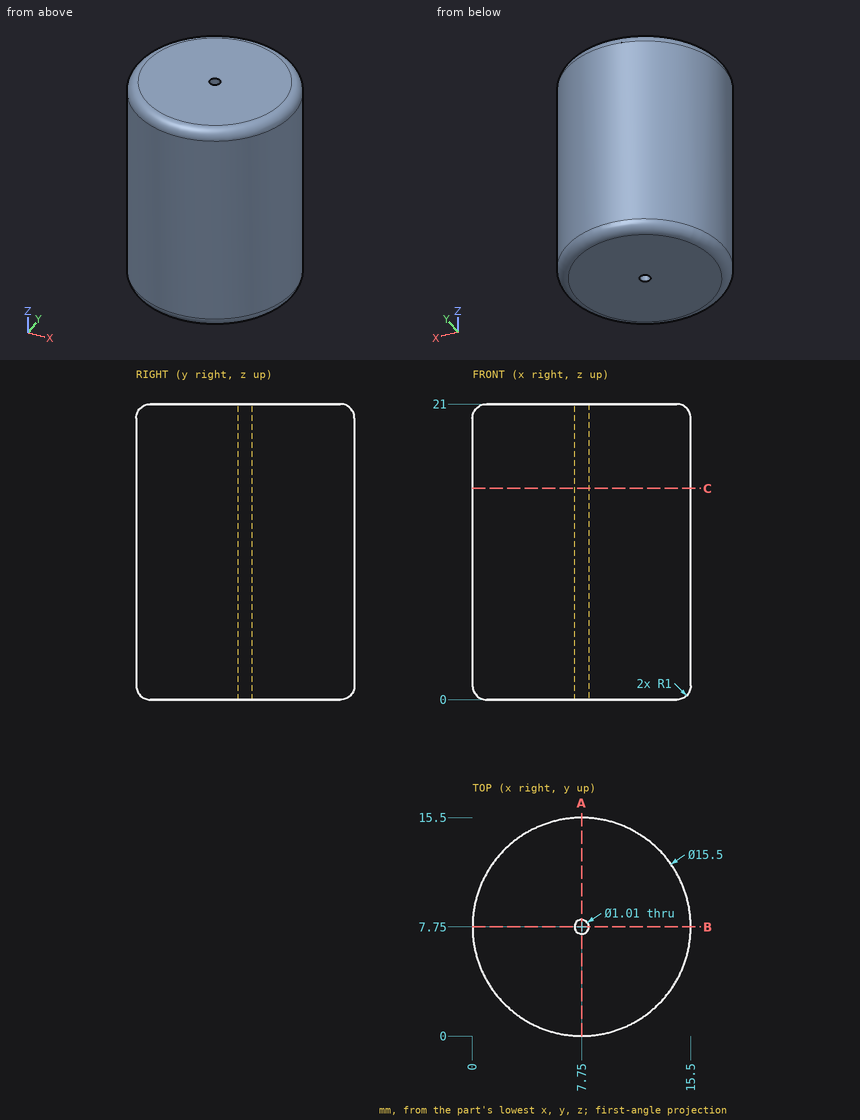
Job drawing, mm, ordinate dimensions from the low corner. One solid piece. Round coordinates to 2 decimals unless told otherwise and drop trailing zeros. Write each loop counter-clockwise with the first axis right and the second up, starting at its lowest first coordinate (ties: lowest second). Pieces come first, ordered by that corner, then holes.
1) Pin check, flat tip, straight feed: pin 1 (3 mm diameter, centred on y = 13, z = 3.5, fed in from +X). Stop position of the tip, or through.
2) Band-saw the part on A-A, the plane x = 7.75. List the corners of the cut face in (y, z) (3 decimals).
3) Drill centre lines: probe 1 along Y at (x, z) = (7.75, 16.5) (3 decimals); probe 2 along X at (y, z) = (10.25, 12.75); probe 3 along Y at (x, z) = (5.5, 5.5). Where is each one in solid material? Low to high.
4) Band-saw the part on C-C, the plane z = 15. List the corners of the cut face in (x, y) (3 decimals), and give its area (3 significant figures).
Ans:
1. pin 1: stops at x = 14.53
2. outline: (0, 1) arc R1 ccw to (1, 0) - (7.245, 0) - (7.245, 21) - (1, 21) arc R1 ccw to (0, 20) - close; (8.255, 0) - (14.5, 0) arc R1 ccw to (15.5, 1) - (15.5, 20) arc R1 ccw to (14.5, 21) - (8.255, 21) - close
3. probe 1: y = 0 to 7.245, 8.255 to 15.5
3. probe 2: x = 0.41 to 15.09
3. probe 3: y = 0.33 to 15.17
4. outline: circle Ø15.5 at (7.75, 7.75); hole circle Ø1.01 at (7.75, 7.75)
4. area: 188 mm2
